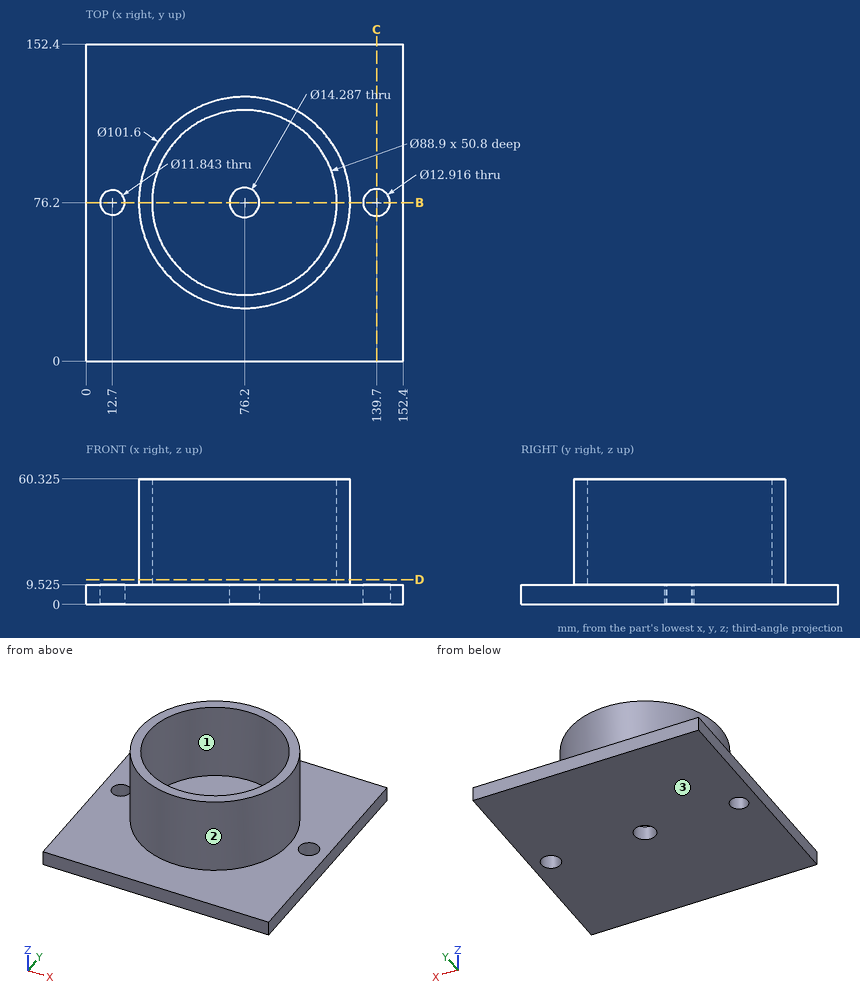
Can you work these out from the drawing? Everything is in mm from the part's minimum corner. Round coordinates to 2 decimals unless told otherwise and drop trailing zeros. Write each loop counter-clockwise with the first axis right and the second up, starting at its lowest first coordinate (ties: lowest second). Pieces come first, ordered by that corner, then holes. Notation, with made-up numbers: (-1, 67) - (14, 67) arc R15 ccw to (14, 77) - close; hole circle Ø2 at (46, 0). An arc over 180 degrees is marked (long way). Use a Markdown table: item, result.
Q1. Thinking about a two-plate mould opening in X: for the marked faces 1, 2 and 3, which applies, released by +X, released by -X, zero draft, split by the parting line, or undercut?
Output values:
| item | result |
|---|---|
| face 1 | undercut |
| face 2 | split by the parting line |
| face 3 | zero draft |
Q2. I want a section at B-B (y = 76.2). Count the separate pieces of the cut face and the enclosed holes in it.
Output values:
| item | result |
|---|---|
| separate pieces | 4 |
| enclosed holes | 0 |
Q3. I want a section at C-C (x = 139.7). List the corners of the cut face in (y, z) for me (1 decimal).
Output values:
| item | result |
|---|---|
| outline | (0, 0) - (69.7, 0) - (69.7, 9.5) - (0, 9.5) - close; (82.7, 0) - (152.4, 0) - (152.4, 9.5) - (82.7, 9.5) - close |
Q4. I want a section at D-D (z = 12). List the corners of the cut face in (x, y) for me, plus the area to 3 significant figures.
Output values:
| item | result |
|---|---|
| outline | circle Ø101.6 at (76.2, 76.2); hole circle Ø88.9 at (76.2, 76.2) |
| area | 1,900 mm2 |
Q5. Please list where these lines run through material, in increasing order: L1, parallel to Y at x = 76.2, z = 36.5; L2, parallel to Y at x = 12.7, z = 2.5; L3, parallel to Z at x = 95, y = 92 (1 decimal).
Output values:
| item | result |
|---|---|
| L1 | 25.4 to 31.75, 120.65 to 127 |
| L2 | 0 to 70.28, 82.12 to 152.4 |
| L3 | 0 to 9.5 |
Q6. For pin 1 (1 mm diameter, centred on x = 44.5, y = 109, fed in from -Z); pin 2 (2 mm diameter, centred on x = 73, z = 37.5, fed in from -Y); pin 3 (5 mm diameter, centred on y = 113, z = 38.5, fed in from +X); pin 4 (10 mm diameter, centred on y = 26, z = 40, fed in from -X) (1 decimal), each with a flat end and sliding along its axis, tell me the tip position at first contact or that it passes through.
Output values:
| item | result |
|---|---|
| pin 1 | z = 0 |
| pin 2 | y = 25.45 |
| pin 3 | x = 113.67 |
| pin 4 | x = 53 |
